Input: dimensioned drawing with shaded views. Units: mm. Origin: part minimum x, y, z. Give positions to 0.01 mm unless a question says otherwise; leave off trailing zeros. Loops run counter-clockwise (first coordinate to the right, second up) from the corner with the lowest first, then second, coordinate; pieces in that order, holes last. Notation, with made-up numbers: M 40,2.5 L 79,2.5 A9 cw 79,10.5 Z; hole C 47.25,22 d10. An arc over 180 degrees is marked long. One line per question, with ' | ' between items. Start each with the question number.
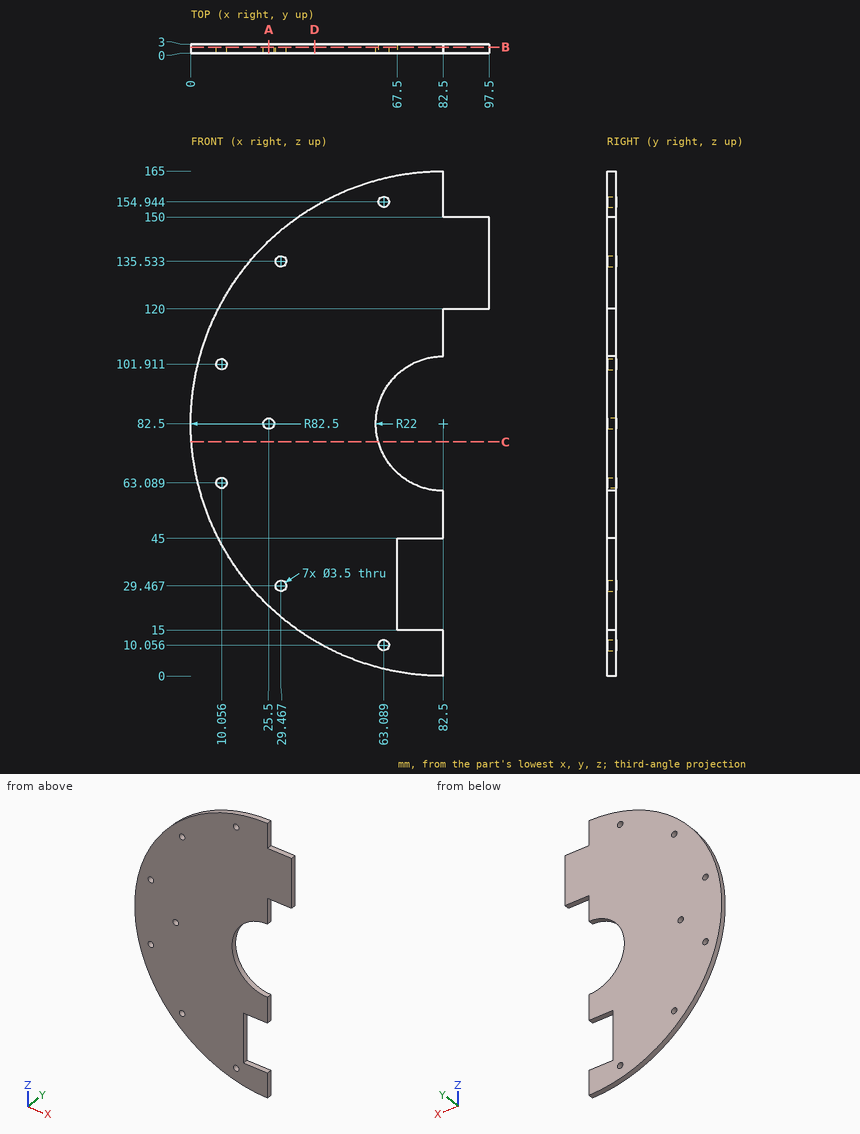
Q1. Contact query for flat-ended pins moving along their axis: pin 1 (1 mm diameter, centred on y = 2, z = 87.5, fed in from +X); pin 2 (2 mm diameter, centred on x = 10.06, z = 101.91, fed in from +Y); pin 3 (0.9 mm diameter, centred on x = 78.5, y = 2, fed in from -Z); pin 4 (1.5 mm diameter, centred on y = 0.5, z = 118.5, fed in from +X). Output: stop coordinate, or through.
Q2. Section D-D, the plane x = 40.5. Output: boundary loops of the cut face in (y, z).
Q3. Material intervals for L1, parallel to Z at x = 71, y = 1.3 (1 decimal); L2, parallel to Z at x = 68.5, y = 1.6 (1 decimal); L3, parallel to Z at x = 90, y = 1.7, sorted ascending.
Q4. Section A-A, the plane x = 25.5. Output: boundary loops of the cut face in (y, z).
Q5. Section B-B, the plane y = 2. Count the separate pieces of the cut face and the enclosed holes in it, plus the area to 3 significant figures.
Q6. Section C-C, the plane z = 76.5. Output: boundary loops of the cut face in (x, y).
Model answer:
1) pin 1: stops at x = 61.2 | pin 2: passes through | pin 3: stops at z = 0.08 | pin 4: stops at x = 82.5
2) outline: M 0,11.49 L 3,11.49 L 3,153.51 L 0,153.51 Z
3) L1: z = 0.8 to 15, 45 to 63.7, 101.3 to 164.2 | L2: z = 1.2 to 15, 45 to 65.5, 99.5 to 163.8 | L3: z = 120 to 150
4) outline: M 0,22.86 L 3,22.86 L 3,80.75 L 0,80.75 Z; M 0,84.25 L 3,84.25 L 3,142.14 L 0,142.14 Z
5) separate pieces: 1 | enclosed holes: 7 | area: 9,860 mm^2
6) outline: M 0.22,0 L 61.33,0 L 61.33,3 L 0.22,3 Z
